from build123d import *

# Parameters (mm, degrees)
F0_W     = 88.9
F0_H     = 38.1
F1_DEPTH = 1752.6
F3_W     = 88.9
F3_H     = 38.1
F3_W_2   = 50.8
F3_H_2   = 19.05
F4_DEPTH = 31.75
F6_DEPTH = 28.576


# Not quite as in the source:
# - a pattern or mirror of a feature is missing from the dataset's text; its kind, count and spacing are read off the source's solid


with BuildPart() as f1:
    # F0 (on Right) → F1 (new body)
    with BuildSketch(Plane.YZ):
        Rectangle(F0_W, F0_H)
    extrude(amount=F1_DEPTH)

    # F3 (on face) → F4 (cut)
    with BuildSketch(Plane(origin=(0, 0, 0), x_dir=(0, -1, 0), z_dir=(-1, 0, 0))):
        Rectangle(F3_W, F3_H)
        Rectangle(F3_W_2, F3_H_2, mode=Mode.SUBTRACT)
    f4 = extrude(amount=-F4_DEPTH, mode=Mode.SUBTRACT)

    # F4_copies: F4 across plane
    add(f4.mirror(Plane(origin=(876.3, 0, 0), x_dir=(0, 0, 1), z_dir=(1, 0, 0))), mode=Mode.SUBTRACT)

    # F5 (on face) → F6 (cut, through all)
    with BuildSketch(Plane.XY.offset(9.525)):
        with BuildLine():
            Line((9.525, 6.35), (9.525, -6.35))
            ThreePointArc((9.525, -6.35), (15.875, -12.7), (22.225, -6.35))
            Line((22.225, -6.35), (22.225, 6.35))
            ThreePointArc((22.225, 6.35), (15.875, 12.7), (9.525, 6.35))
        make_face()
    f6 = extrude(amount=-F6_DEPTH, mode=Mode.SUBTRACT)

    # F6_copies: F6 across plane
    add(f6.mirror(Plane(origin=(876.3, 0, 0), x_dir=(0, 0, 1), z_dir=(1, 0, 0))), mode=Mode.SUBTRACT)


solid = f1.part
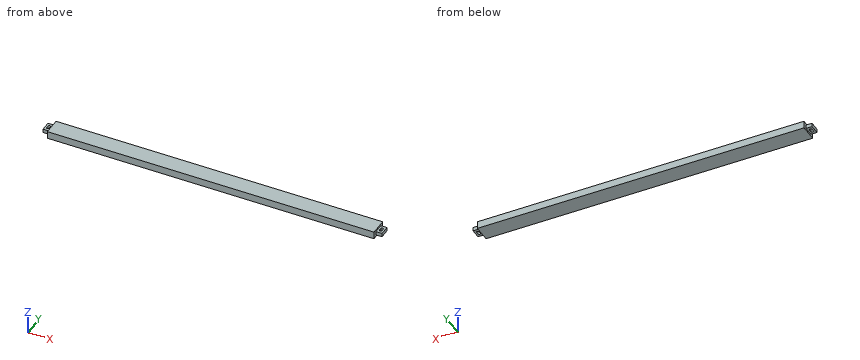
CAD build for the part. Positions are in the model's coordinates, mm. Round coordinates to 2 decimals unless told otherwise and drop trailing zeros. Loops run counter-clockwise (first coordinate to the right, second up) from the corner with the lowest first, then second, coordinate; pieces in that order, holes last.
(1) Drop flat-ended pins along their axis: pin 1 (9.5 mm diameter, centred on x = 1736.5, z = -2, fed in from -Y); pin 2 (2 mm diameter, centred on y = -32, z = 1, fed in from -X); pin 3 (15 mm diameter, centred on x = 9.5, z = 0, fed in from +Y). Give the stop position or say it passes through.
(2) Cut at A-A (z = 3). Give the cut face in (x, y) (3 decimals).
(3) Wall check: line 1 along X through (y, z) = (38.5, -1.5); line 2 along X through (y, z) = (10, -5.5). Give the ranges that are in metal, low to high.
Findings below:
1. pin 1: stops at y = -25.4
1. pin 2: stops at x = 31.75
1. pin 3: stops at y = 25.4
2. outline: (0, -25.4) - (31.75, -25.4) - (31.75, -44.45) - (1720.85, -44.45) - (1720.85, -25.4) - (1752.6, -25.4) - (1752.6, 25.4) - (1720.85, 25.4) - (1720.85, 44.45) - (31.75, 44.45) - (31.75, 25.4) - (0, 25.4) - close; hole (9.525, -6.35) arc R6.35 ccw to (22.225, -6.35) - (22.225, 6.35) arc R6.35 ccw to (9.525, 6.35) - close; hole (1730.375, -6.35) arc R6.35 ccw to (1743.075, -6.35) - (1743.075, 6.35) arc R6.35 ccw to (1730.375, 6.35) - close
3. line 1: x = 31.75 to 1720.85
3. line 2: x = 0 to 10.68, 21.07 to 1731.53, 1741.92 to 1752.6
